Autodesk Inventor part; units mm, degrees
ref_plane "YZ Plane" through (0, 0, 0) normal (1, 0, 0) x (0, 1, 0)
ref_plane "XZ Plane" through (0, 0, 0) normal (0, 1, 0) x (-1, 0, 0)
ref_plane "XY Plane" through (0, 0, 0) normal (0, 0, 1) x (1, 0, 0)
sketch "Sketch1" plane through (0, 0, 0) normal (0, 0, 1) x (1, 0, 0)
  circle A0 centre (0, 0) radius 4
  dimension "d0" = 8
extrude "Extrusion1" add sketch "Sketch1" along normal blind 60.6
chamfer "Chamfer1" distance 0.5 angle 45 2 edges at (-4, 0, 0) (-4, 0, 60.6)
hole "Hole1" at (0, 0, 0) direction (0, 0, 1) diameter 3.242 end through all
properties part number "asjes" material "Aluminum 6061"
Verification items for the finished model (mm, model axes). Coordinates: 2 decimals unless noted, no trailing zeros. Order: outer loops, then holes, each group sorted by start corner. A loop starts at its lowest first (then second) coordinate and runs counter-clockwise, first axis right, second up. Notation, with made-up numbers: (-39, 47.25) -> (-35, 47.25) arc R28 cw to (-35, 70.25) -> close; hole circle Ø3 at (52, -5.75). An arc over 180 degrees is marked (long way). Use CSV: the item, a comma, the result in double quotes. Start each with the question number.
Q1. Section check A-A, the plane y = 0. Record the cut outline in (x, z), and give its area (3 significant figures).
Q2. Section check C-C, the plane z = 42. Record the cut outline in (x, y), and give its area (3 significant figures).
Q3. Draft check along X on faces 1 (the flat face through (1, -2, 60.6)), 2 (the cylindrical face through (-0.867, 3.905, 29.883)), 3 (the cylindrical face through (1.438, 0.748, 30.724)). Enter one of: +X half, -X half, draft (parallel to the pull), parting line (faces both ways), or undercut.
Q4. Thickness scan on line 1 along Y through (x, z) = (0, 14.5); line 2 along Y through (x, z) = (-1, 18.5). Record the ranges inside material, lowest first.
Q5. Depth check by flat-ended pin: P1, Ø1.5, axis at x = 2, z = 23.5, coming from the -Y side; P2, Ø1, axis at x = -3, z = 8.5, coming from the +Y side; P3, Ø2, axis at x = -3, z = 31.5, coming from the -Y side. Enter the tip coordinate at first touch or a pass-through.
Returned:
1,outline,"(-4, 0.5) -> (-3.5, 0) -> (-1.62, 0) -> (-1.62, 60.6) -> (-3.5, 60.6) -> (-4, 60.1) -> close; (1.62, 0) -> (3.5, 0) -> (4, 0.5) -> (4, 60.1) -> (3.5, 60.6) -> (1.62, 60.6) -> close"
1,area,"288 mm^2"
2,outline,"circle Ø8 at (0, 0); hole circle Ø3.24 at (0, 0)"
2,area,"42.0 mm^2"
3,face 1,"draft"
3,face 2,"parting line"
3,face 3,"undercut"
4,line 1,"y = -4 to -1.62, 1.62 to 4"
4,line 2,"y = -3.87 to -1.28, 1.28 to 3.87"
5,P1,"stops at y = -3.8"
5,P2,"stops at y = 3.12"
5,P3,"stops at y = -3.46"
